Can you work these out from the model? Positions are in its coordinate system, mm. Round coordinates to 2 decimals unless told otherwise and drop trailing zeros. Write item = value, one per line.
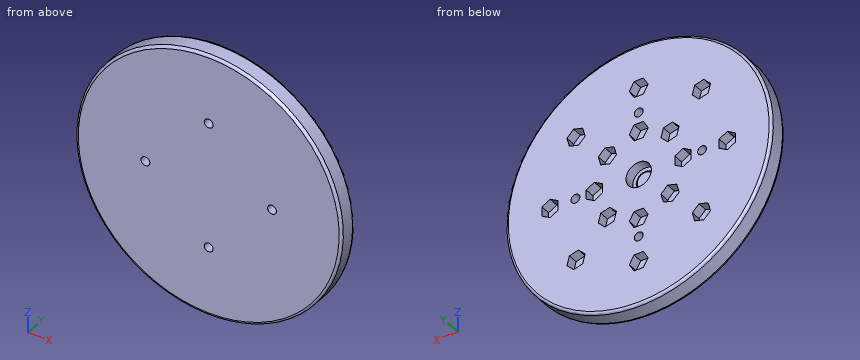
from build123d import *

# Parameters (mm, degrees)
SKETCH1_R                 = 105
BOSS_EXTRUDE1_DEPTH       = 7.5
SKETCH2_R                 = 3.5
CUT_EXTRUDE2_DEPTH        = 7.5
CIRPATTERN1_COUNT         = 2
CIRPATTERN1_ANGLE         = 90
FILLET2_R                 = 2
CUT_EXTRUDE3_DEPTH        = 8
LPATTERN1_COUNT           = 3
LPATTERN1_PITCH           = 35
CIRPATTERN2_COUNT         = 8
CIRPATTERN2_COPY_1_DEPTH  = 8
CIRPATTERN2_COPY_2_DEPTH  = 8
CIRPATTERN2_COPY_3_DEPTH  = 8
CIRPATTERN2_COPY_4_DEPTH  = 8
CIRPATTERN2_COPY_5_DEPTH  = 8
CIRPATTERN2_COPY_6_DEPTH  = 8
CIRPATTERN2_COPY_7_DEPTH  = 8
CIRPATTERN2_COPY_8_DEPTH  = 8
CIRPATTERN2_COPY_9_DEPTH  = 8
CIRPATTERN2_COPY_10_DEPTH = 8
CIRPATTERN2_COPY_11_DEPTH = 8
CIRPATTERN2_COPY_12_DEPTH = 8
CIRPATTERN2_COPY_13_DEPTH = 8
CIRPATTERN2_COPY_14_DEPTH = 8
SKETCH4_R                 = 10
CUT_EXTRUDE4_DEPTH        = 8


with BuildPart() as part:
    # Sketch1 → Boss-Extrude1 (new, symmetric)
    with BuildSketch(Plane(origin=(0, 0, 0), x_dir=(1, 0, 0), z_dir=(0, 1, 0))):
        with Locations(Location((0, 0, 0), (0, 0, 270))):
            Circle(SKETCH1_R)
    extrude(amount=BOSS_EXTRUDE1_DEPTH, both=True)

    # Sketch2 → Cut-Extrude2 (cut, symmetric)
    with BuildSketch(Plane(origin=(0, 0, 0), x_dir=(1, 0, 0), z_dir=(0, 1, 0))):
        with Locations(Location((0, 50, 0), (0, 0, 270))):
            Circle(SKETCH2_R)
        with Locations(Location((0, -50, 0), (0, 0, 270))):
            Circle(SKETCH2_R)
    cut_extrude2 = extrude(amount=CUT_EXTRUDE2_DEPTH, both=True, mode=Mode.SUBTRACT)

    # CirPattern1: Cut-Extrude2 ×2 about axis
    cirpattern1_axis = Axis((0, 0, 0), (0, 1, 0))
    for i in range(1, CIRPATTERN1_COUNT):
        add(cut_extrude2.rotate(cirpattern1_axis, i * CIRPATTERN1_ANGLE / (CIRPATTERN1_COUNT - 1)), mode=Mode.SUBTRACT)

    # Fillet2
    fillet2_edges = [part.edges().sort_by_distance(p)[0] for p in [
        (0, -7.5, -105),
        (0, 7.5, -105),
    ]]
    fillet(fillet2_edges, radius=FILLET2_R)

    # Sketch3 → Cut-Extrude3 (cut)
    with BuildSketch(Plane(origin=(0, 7.5, 0), x_dir=(1, 0, 0), z_dir=(0, 1, 0))):
        Polygon((3.718255526, 6.440207487), (-3.718255526, 6.440207487), (-7.436511052, 0), (-3.718255526, -6.440207487), (3.718255526, -6.440207487), (7.436511052, 0), align=None)
    cut_extrude3 = extrude(amount=-CUT_EXTRUDE3_DEPTH, mode=Mode.SUBTRACT)

    # LPattern1: Cut-Extrude3 ×3
    with Locations(*[(0, 0, i * LPATTERN1_PITCH) for i in range(1, LPATTERN1_COUNT)]):
        add(cut_extrude3, mode=Mode.SUBTRACT)

    # CirPattern2: Cut-Extrude3 ×8 about axis
    cirpattern2_axis = Axis((0, 0, 0), (0, 1, 0))
    for i in range(1, CIRPATTERN2_COUNT):
        add(cut_extrude3.rotate(cirpattern2_axis, i * 360 / CIRPATTERN2_COUNT), mode=Mode.SUBTRACT)

    # CirPattern2 copy 1 sketch → CirPattern2 copy 1 (cut)
    with BuildSketch(Plane(origin=(24.748737342, 7.5, 24.748737342), x_dir=(0.7071067811865476, 0, -0.7071067811865475), z_dir=(0, 1, 0))):
        Polygon((3.718255526, 6.440207487), (-3.718255526, 6.440207487), (-7.436511052, 0), (-3.718255526, -6.440207487), (3.718255526, -6.440207487), (7.436511052, 0), align=None)
    extrude(amount=-CIRPATTERN2_COPY_1_DEPTH, mode=Mode.SUBTRACT)

    # CirPattern2 copy 2 sketch → CirPattern2 copy 2 (cut)
    with BuildSketch(Plane(origin=(35, 7.5, 0), x_dir=(0, 0, -1), z_dir=(0, 1, 0))):
        Polygon((3.718255526, 6.440207487), (-3.718255526, 6.440207487), (-7.436511052, 0), (-3.718255526, -6.440207487), (3.718255526, -6.440207487), (7.436511052, 0), align=None)
    extrude(amount=-CIRPATTERN2_COPY_2_DEPTH, mode=Mode.SUBTRACT)

    # CirPattern2 copy 3 sketch → CirPattern2 copy 3 (cut)
    with BuildSketch(Plane(origin=(24.748737342, 7.5, -24.748737342), x_dir=(-0.7071067811865475, 0, -0.7071067811865476), z_dir=(0, 1, 0))):
        Polygon((3.718255526, 6.440207487), (-3.718255526, 6.440207487), (-7.436511052, 0), (-3.718255526, -6.440207487), (3.718255526, -6.440207487), (7.436511052, 0), align=None)
    extrude(amount=-CIRPATTERN2_COPY_3_DEPTH, mode=Mode.SUBTRACT)

    # CirPattern2 copy 4 sketch → CirPattern2 copy 4 (cut)
    with BuildSketch(Plane(origin=(0, 7.5, -35), x_dir=(-1, 0, 0), z_dir=(0, 1, 0))):
        Polygon((3.718255526, 6.440207487), (-3.718255526, 6.440207487), (-7.436511052, 0), (-3.718255526, -6.440207487), (3.718255526, -6.440207487), (7.436511052, 0), align=None)
    extrude(amount=-CIRPATTERN2_COPY_4_DEPTH, mode=Mode.SUBTRACT)

    # CirPattern2 copy 5 sketch → CirPattern2 copy 5 (cut)
    with BuildSketch(Plane(origin=(-24.748737342, 7.5, -24.748737342), x_dir=(-0.7071067811865477, 0, 0.7071067811865475), z_dir=(0, 1, 0))):
        Polygon((3.718255526, 6.440207487), (-3.718255526, 6.440207487), (-7.436511052, 0), (-3.718255526, -6.440207487), (3.718255526, -6.440207487), (7.436511052, 0), align=None)
    extrude(amount=-CIRPATTERN2_COPY_5_DEPTH, mode=Mode.SUBTRACT)

    # CirPattern2 copy 6 sketch → CirPattern2 copy 6 (cut)
    with BuildSketch(Plane(origin=(-35, 7.5, 0), x_dir=(0, 0, 1), z_dir=(0, 1, 0))):
        Polygon((3.718255526, 6.440207487), (-3.718255526, 6.440207487), (-7.436511052, 0), (-3.718255526, -6.440207487), (3.718255526, -6.440207487), (7.436511052, 0), align=None)
    extrude(amount=-CIRPATTERN2_COPY_6_DEPTH, mode=Mode.SUBTRACT)

    # CirPattern2 copy 7 sketch → CirPattern2 copy 7 (cut)
    with BuildSketch(Plane(origin=(-24.748737342, 7.5, 24.748737342), x_dir=(0.7071067811865474, 0, 0.7071067811865477), z_dir=(0, 1, 0))):
        Polygon((3.718255526, 6.440207487), (-3.718255526, 6.440207487), (-7.436511052, 0), (-3.718255526, -6.440207487), (3.718255526, -6.440207487), (7.436511052, 0), align=None)
    extrude(amount=-CIRPATTERN2_COPY_7_DEPTH, mode=Mode.SUBTRACT)

    # CirPattern2 copy 8 sketch → CirPattern2 copy 8 (cut)
    with BuildSketch(Plane(origin=(49.497474683, 7.5, 49.497474683), x_dir=(0.7071067811865476, 0, -0.7071067811865475), z_dir=(0, 1, 0))):
        Polygon((3.718255526, 6.440207487), (-3.718255526, 6.440207487), (-7.436511052, 0), (-3.718255526, -6.440207487), (3.718255526, -6.440207487), (7.436511052, 0), align=None)
    extrude(amount=-CIRPATTERN2_COPY_8_DEPTH, mode=Mode.SUBTRACT)

    # CirPattern2 copy 9 sketch → CirPattern2 copy 9 (cut)
    with BuildSketch(Plane(origin=(70, 7.5, 0), x_dir=(0, 0, -1), z_dir=(0, 1, 0))):
        Polygon((3.718255526, 6.440207487), (-3.718255526, 6.440207487), (-7.436511052, 0), (-3.718255526, -6.440207487), (3.718255526, -6.440207487), (7.436511052, 0), align=None)
    extrude(amount=-CIRPATTERN2_COPY_9_DEPTH, mode=Mode.SUBTRACT)

    # CirPattern2 copy 10 sketch → CirPattern2 copy 10 (cut)
    with BuildSketch(Plane(origin=(49.497474683, 7.5, -49.497474683), x_dir=(-0.7071067811865475, 0, -0.7071067811865476), z_dir=(0, 1, 0))):
        Polygon((3.718255526, 6.440207487), (-3.718255526, 6.440207487), (-7.436511052, 0), (-3.718255526, -6.440207487), (3.718255526, -6.440207487), (7.436511052, 0), align=None)
    extrude(amount=-CIRPATTERN2_COPY_10_DEPTH, mode=Mode.SUBTRACT)

    # CirPattern2 copy 11 sketch → CirPattern2 copy 11 (cut)
    with BuildSketch(Plane(origin=(0, 7.5, -70), x_dir=(-1, 0, 0), z_dir=(0, 1, 0))):
        Polygon((3.718255526, 6.440207487), (-3.718255526, 6.440207487), (-7.436511052, 0), (-3.718255526, -6.440207487), (3.718255526, -6.440207487), (7.436511052, 0), align=None)
    extrude(amount=-CIRPATTERN2_COPY_11_DEPTH, mode=Mode.SUBTRACT)

    # CirPattern2 copy 12 sketch → CirPattern2 copy 12 (cut)
    with BuildSketch(Plane(origin=(-49.497474683, 7.5, -49.497474683), x_dir=(-0.7071067811865477, 0, 0.7071067811865475), z_dir=(0, 1, 0))):
        Polygon((3.718255526, 6.440207487), (-3.718255526, 6.440207487), (-7.436511052, 0), (-3.718255526, -6.440207487), (3.718255526, -6.440207487), (7.436511052, 0), align=None)
    extrude(amount=-CIRPATTERN2_COPY_12_DEPTH, mode=Mode.SUBTRACT)

    # CirPattern2 copy 13 sketch → CirPattern2 copy 13 (cut)
    with BuildSketch(Plane(origin=(-70, 7.5, 0), x_dir=(0, 0, 1), z_dir=(0, 1, 0))):
        Polygon((3.718255526, 6.440207487), (-3.718255526, 6.440207487), (-7.436511052, 0), (-3.718255526, -6.440207487), (3.718255526, -6.440207487), (7.436511052, 0), align=None)
    extrude(amount=-CIRPATTERN2_COPY_13_DEPTH, mode=Mode.SUBTRACT)

    # CirPattern2 copy 14 sketch → CirPattern2 copy 14 (cut)
    with BuildSketch(Plane(origin=(-49.497474683, 7.5, 49.497474683), x_dir=(0.7071067811865474, 0, 0.7071067811865477), z_dir=(0, 1, 0))):
        Polygon((3.718255526, 6.440207487), (-3.718255526, 6.440207487), (-7.436511052, 0), (-3.718255526, -6.440207487), (3.718255526, -6.440207487), (7.436511052, 0), align=None)
    extrude(amount=-CIRPATTERN2_COPY_14_DEPTH, mode=Mode.SUBTRACT)

    # Sketch4 → Cut-Extrude4 (cut)
    with BuildSketch(Plane(origin=(0, 7.5, 0), x_dir=(1, 0, 0), z_dir=(0, 1, 0))):
        with Locations(Location((0, 0, 0), (0, 0, 270))):
            Circle(SKETCH4_R)
    extrude(amount=-CUT_EXTRUDE4_DEPTH, mode=Mode.SUBTRACT)


solid = part.part
1. Suppose I cut it at A-A, the plane y = 3. Count the separate pieces of the cut face and the enclosed holes in it, and give its area (3 significant figures).
Entries:
separate_pieces = 1
enclosed_holes = 21
area = 31,900 mm²
2. I need wall thicknesses on line 1 (Y direction, x = 4.5, z = 73.5); line 2 (X direction, y = 3.5, z = 50); line 3 (X direction, y = -4, z = -50). Which ranges of each line are inside material? Lowest first, please. Write a range as [from, to].
Entries:
line_1 = [-7.5, -0.5]
line_2 = [-92.33, -56.3], [-42.96, -3.5], [3.5, 42.96], [56.3, 92.33]
line_3 = [-92.33, -3.5], [3.5, 92.33]
3. I'm going to push flat-ended pins straight in: pin 1 (8 mm diameter, centred on x = 8.5, y = -1, fed in from -Z); pin 2 (10 mm diameter, centred on x = -46, z = 48, fed in from +Y); pin 3 (1.5 mm diameter, centred on y = -0.5, z = 59, fed in from +X); pin 4 (1.5 mm diameter, centred on x = -9.5, y = 3.5, fed in from +Z). Where does each tip first touch, or does it pass through?
Entries:
pin_1 = -104.9
pin_2 = 7.5
pin_3 = 87.36
pin_4 = 104.63
